```python
from build123d import *

# Parameters (mm, degrees)
F1_DEPTH    = 25.4
F2_R        = 11.0950895879
F2_R_2      = 11.0767516797
F3_DEPTH    = 51.816
F5_DEPTH    = 12.7
F6_T1_DEPTH = 77.7777149491
F6_T3_DEPTH = 77.7777149491
F7_R        = 5.3247390171
F8_DEPTH    = 189.484


# Not quite as in the source:
# - a fillet or chamfer that OpenCascade refuses, or shapes differently, is made with other operations: its cross-section is extruded or revolved along the edge and cut away or added


with BuildPart() as f1:
    # F0 (on Top) → F1 (new body)
    with BuildSketch(Plane.XY):
        with BuildLine():
            Line((-84.3394622207, -22.0487453043), (-84.3394622207, 25.6632901728))
            ThreePointArc((-84.3394622207, 25.6632901728), (-109.0315538503, 1.8072724342), (-84.3394622207, -22.0487453043))
        make_face()
        Polygon((83.375572493, 25.6632901728), (-84.3394622207, 25.6632901728), (-84.3394622207, -22.0487453043), (83.375572493, -22.0487453043), (84.8214030266, -22.0487453043), (84.8214030266, 25.6632901728), align=None)
        with BuildLine():
            ThreePointArc((84.8214030266, -22.0487453043), (107.965456332, 1.8072724342), (84.8214030266, 25.6632901728))
            Line((84.8214030266, 25.6632901728), (84.8214030266, -22.0487453043))
        make_face()
    extrude(amount=F1_DEPTH)

    # F2 (on face) → F3 (cut)
    with BuildSketch(Plane.XY.offset(25.4)):
        with Locations((-76.1863589287, 0)):
            Circle(F2_R)
        with Locations((76.3475745916, 0)):
            Circle(F2_R_2)
    extrude(amount=-F3_DEPTH, mode=Mode.SUBTRACT)

    # F4 (on Front) → F5 (join, symmetric)
    with BuildSketch(Plane.XZ):
        with BuildLine():
            Line((-34.8596895088, 72.9802176356), (-48.2503287494, 72.9802176356))
            Line((-48.2503287494, 72.9802176356), (-48.2503287494, 0))
            Line((-48.2503287494, 0), (48.2503287494, 0))
            Line((48.2503287494, 0), (48.2503287494, 72.9802176356))
            Line((48.2503287494, 72.9802176356), (34.8596895088, 72.9802176356))
            ThreePointArc((34.8596895088, 72.9802176356), (0, 38.1205281268), (-34.8596895088, 72.9802176356))
        make_face()
    extrude(amount=F5_DEPTH, both=True)

    # F6: fillet of radius 12.8774151417 on 4 edges, made by hand

    # F6_s2 → F6_t1 (cut)
    with BuildSketch(Plane.YZ.offset(-80.4438666037)):
        with BuildLine():
            ThreePointArc((-12.7, 60.1028024939), (-8.9282924292, 69.2085100648), (0.1774151417, 72.9802176356))
            Line((0.1774151417, 72.9802176356), (-12.7, 72.9802176356))
            Line((-12.7, 72.9802176356), (-12.7, 60.1028024939))
        make_face()
        with BuildLine():
            ThreePointArc((12.7, 60.1028024939), (8.9282924292, 69.2085100648), (-0.1774151417, 72.9802176356))
            Line((-0.1774151417, 72.9802176356), (12.7, 72.9802176356))
            Line((12.7, 72.9802176356), (12.7, 60.1028024939))
        make_face()
    extrude(amount=F6_T1_DEPTH, mode=Mode.SUBTRACT)

    # F6_s4 → F6_t3 (cut)
    with BuildSketch(Plane.YZ.offset(2.6661516546)):
        with BuildLine():
            ThreePointArc((12.7, 60.1028024939), (8.9282924292, 69.2085100648), (-0.1774151417, 72.9802176356))
            Line((-0.1774151417, 72.9802176356), (12.7, 72.9802176356))
            Line((12.7, 72.9802176356), (12.7, 60.1028024939))
        make_face()
        with BuildLine():
            ThreePointArc((-12.7, 60.1028024939), (-8.9282924292, 69.2085100648), (0.1774151417, 72.9802176356))
            Line((0.1774151417, 72.9802176356), (-12.7, 72.9802176356))
            Line((-12.7, 72.9802176356), (-12.7, 60.1028024939))
        make_face()
    extrude(amount=F6_T3_DEPTH, mode=Mode.SUBTRACT)

    # F7 (on face) → F8 (cut)
    with BuildSketch(Plane(origin=(-48.2503287494, 0, 0), x_dir=(0, -1, 0), z_dir=(-1, 0, 0))):
        with Locations((0.1774151417, 60.1028024939)):
            Circle(F7_R)
    extrude(amount=-F8_DEPTH, mode=Mode.SUBTRACT)


solid = f1.part
```
Check sheet for the modelled part. Datum: model origin and axes. Units: mm. A direction names the side the tool comes from. Give positions to 0.01 mm unless a question says otherwise; leave off trailing zeros. Write each loop counter-clockwise with the first axis right and the second up, starting at its lowest first coordinate (ties: lowest second). Pieces come first, ordered by that corner, then holes.
Item 1: Cross-section at A-A (z = 18). Enter the section's corners in (x, y), and give its area (3 significant figures).
Item 2: Draft check along Z on faces 5 (the face through (-2, 2, 0)), 6 (the face through (-40.433, -9.089, 69.045)), 7 (the face through (40.917, 0.977, 54.905)), 8 (the face through (65.28, 0.49, 12.88)). Enter one of: released by +Z, released by -Z, zero draft, split by the parting line, or undercut.
Item 3: Cross-section at B-B (x = 0). Enter the section's corners in (y, z).
Item 4: Cross-section at D-D (z = 62.5). Enter the section's corners in (x, y), and give its area (3 significant figures).
Item 5: Scan lines: L1, parallel to Y at x = -47.5, z = 52; L2, parallel to Y at x = 39, z = 11.5; L3, parallel to X at y = -7, z = 13. Record each from-to range of solid material in increasing order.
Item 6: Cross-section at C-C (y = -8). Enter the section's corners in (x, z).
Item 7: Access from +Z, -Z, +X, -X, +Y, -Y to the whole of each face (thin tool, end or side, straight path). Record for faces 1 (the face through (-48.25, 0, 50)), 2 (the face through (-1, -12.7, 35)), 3 (the face through (-1, 12.7, 35)), 4 (the face through (48.25, 0, 49)).
Item 8: Gauge pin test, flat ends, axial feed: pin 1 (6 mm diameter, centred on y = -2, z = 39.5, fed in from +X); pin 2 (12.5 mm diameter, centred on y = -5, z = 55.5, fed in from -X); pin 3 (10 mm diameter, centred on x = -50.5, z = 56, fed in from -Y). Record the tip position at first contact, or that the pin passes through.
Report:
1. outline: (-84.34, -22.05) - (84.82, -22.05) arc R23.87 ccw to (84.82, 25.66) - (-84.34, 25.66) arc R23.87 ccw (long way) to start; hole circle Ø22.19 at (-76.19, 0); hole circle Ø22.15 at (76.35, 0)
1. area: 9,090 mm2
2. face 5: released by -Z
2. face 6: released by +Z
2. face 7: undercut
2. face 8: zero draft
3. outline: (-22.05, 0) - (25.66, 0) - (25.66, 25.4) - (12.7, 25.4) - (12.7, 38.12) - (-12.7, 38.12) - (-12.7, 25.4) - (-22.05, 25.4) - close
4. outline: (-48.25, -12.47) - (-33.25, -12.47) - (-33.25, -4.93) - (-48.25, -4.93) - close; (-48.25, 4.58) - (-33.25, 4.58) - (-33.25, 12.47) - (-48.25, 12.47) - close; (33.25, -12.47) - (48.25, -12.47) - (48.25, -4.93) - (33.25, -4.93) - close; (33.25, 4.58) - (48.25, 4.58) - (48.25, 12.47) - (33.25, 12.47) - close
4. area: 463 mm2
5. L1: y = -12.7 to 12.7
5. L2: y = -22.05 to 25.66
5. L3: x = -107.35 to -84.79, -67.58 to 67.76, 84.93 to 106.28
6. outline: (-106.92, 0) - (-83.87, 0) - (-83.87, 25.4) - (-106.92, 25.4) - close; (-68.5, 0) - (68.69, 0) - (68.69, 25.4) - (48.25, 25.4) - (48.25, 70.05) - (34.74, 70.05) arc R34.86 cw to (-34.74, 70.05) - (-48.25, 70.05) - (-48.25, 25.4) - (-68.5, 25.4) - close; (84.01, 0) - (105.86, 0) - (105.86, 25.4) - (84.01, 25.4) - close
7. face 1: +Z, -X, +Y, -Y
7. face 2: +Z, +X, -X, -Y
7. face 3: +Z, +X, -X, +Y
7. face 4: +Z, +X, +Y, -Y
8. pin 1: stops at x = 48.25
8. pin 2: stops at x = -48.25
8. pin 3: stops at y = -12.7
